Autodesk Inventor part; units mm, degrees
ref_plane "YZ Plane" through (0, 0, 0) normal (1, 0, 0) x (0, 1, 0)
ref_plane "XZ Plane" through (0, 0, 0) normal (0, 1, 0) x (-1, 0, 0)
ref_plane "XY Plane" through (0, 0, 0) normal (0, 0, 1) x (1, 0, 0)
sketch "Sketch1" plane through (0, 0, 0) normal (0, 1, 0) x (-1, 0, 0)
  line L0 (0, 0) -> (12.3, 0)
  line L1 (12.3, 0) -> (12.3, 15)
  line L2 (12.3, 15) -> (0, 15)
  line L3 (0, 15) -> (0, 0)
  dimension "d0" = 15
  dimension "d1" = 12.3
extrude "Extrusion1" add sketch "Sketch1" along normal mid plane 65
sketch "Sketch2" plane through (-12.3, -32.5, 15) normal (-1, 0, 0) x (0, 0, 1)
  circle A0 centre (-7.5, 7.5) radius 3.25
  circle A1 centre (-7.5, 57.5) radius 3.25
  circle A2 centre (-7.5, 7.5) radius 5.5
  circle A3 centre (-7.5, 57.5) radius 5.5
  line L0 (0, 0) -> (-15, 0)
  line L1 (-15, 32.5) -> (12.3047, 32.5) construction
  dimension "d4" = 6.5
  dimension "d5" = 6.5
  dimension "d8" = 11
  dimension "d9" = 11
  dimension "d26" = 25
  dimension "d27" = 25
extrude "Extrusion2" cut sketch "Sketch2" against normal through all contours A0 | A1
extrude "Extrusion3" cut sketch "Sketch2" against normal blind 21.3
sketch "Sketch3" plane through (-12.3, -32.5, 15) normal (-1, 0, 0) x (0, 0, 1)
  circle A0 centre (-7.5, 16.395) radius 3
  line L0 (0, 0) -> (-15, 0)
  circle A1 centre (-7.5, 41.395) radius 3
  point P0 (-15, 32.5)
  dimension "d14" = 6
  dimension "d22" = 16.395
  dimension "d23" = 6
  dimension "d24" = 25
hole "Hole1" at (-12.3, -16.105, 7.5) at (-12.3, 8.895, 7.5) direction (1, 0, 0) diameter 4.917 depth 15.1 tip angle 118
sketch "Sketch4" plane through (-12.3, -32.5, 15) normal (-1, 0, 0) x (0, 0, 1)
  point P0 (-15, 32.5)
properties part number "HeadbarHolderBracket_v2" material "Aluminum 6061"
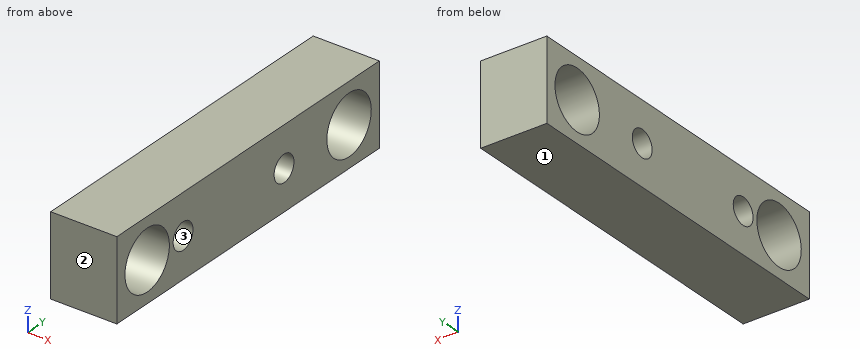
Check sheet for the modelled part. Datum: model origin and axes. Units: mm. Face numbers are marked on the shaded views. Give positions to 0.01 mm unless a question says otherwise; leave off trailing zeros. Order: outer loops, then holes, each group sorted by start corner. A loop starts at its lowest first (then second) coordinate and runs counter-clockwise, first axis right, second up. Notation, with made-up numbers: M 74,84.5 L 94,84.5 A17 cw 94,101.5 Z; hole C -4,85.5 d2. An arc over 180 degrees is marked long. Answer as CSV lines item,"result". Start each with the question number.
Item 1: Thickness scan on line 1 (Y direction, x = -9.5, z = 7.5); line 2 (Y direction, x = -10.5, z = 12.25); line 3 (Y direction, x = -2.5, z = 5.75). Record the ranges inside material, lowest first. Write a range as [from, to].
Item 2: Cross-section at A-A on z = 7.5. Enter the section's corners in (x, y).
Item 3: Cross-section at C-C on z = 11.5. Enter the section's corners in (x, y).
Item 4: Cross-section at D-D on x = -2. Enter the section's corners in (y, z) (1 decimal), plus the area to 3 significant figures.
Item 5: Mould release check, pull along Y, two halves, no side actions. Record for the marked faces 1, 2 and 3: +Y half, -Y half, draft (parallel to the pull), parting line (faces both ways), or undercut.
Item 6: Cross-section at B-B on y = 25. Enter the section's corners in (x, z).
Established:
1,line 1,"y = [-32.5, -30.5], [-19.5, -18.56], [-13.65, 6.44], [11.35, 19.5], [30.5, 32.5]"
1,line 2,"y = [-32.5, -27.77], [-22.23, 22.23], [27.77, 32.5]"
1,line 3,"y = [-32.5, -30.21], [-19.79, -17.83], [-14.38, 7.17], [10.62, 19.79], [30.21, 32.5]"
2,outline,"M -12.3,-32.5 L 0,-32.5 L 0,-30.5 L -12.3,-30.5 Z; M -12.3,-19.5 L 0,-19.5 L 0,-18.56 L -12.3,-18.56 Z; M -12.3,-13.65 L 0,-13.65 L 0,6.44 L -12.3,6.44 Z; M -12.3,11.35 L 0,11.35 L 0,19.5 L -12.3,19.5 Z; M -12.3,30.5 L 0,30.5 L 0,32.5 L -12.3,32.5 Z"
3,outline,"M -12.3,-32.5 L 0,-32.5 L 0,-28.77 L -12.3,-28.77 Z; M -12.3,-21.23 L 0,-21.23 L 0,21.23 L -12.3,21.23 Z; M -12.3,28.77 L 0,28.77 L 0,32.5 L -12.3,32.5 Z"
4,outline,"M -32.5,0 L 32.5,0 L 32.5,15 L -32.5,15 Z; hole C -25,7.5 d11; hole C -16.1,7.5 d4.9; hole C 8.9,7.5 d4.9; hole C 25,7.5 d11"
4,area,"747 mm^2"
5,face 1,"draft"
5,face 2,"-Y half"
5,face 3,"undercut"
6,outline,"M -12.3,0 L 0,0 L 0,2 L -12.3,2 Z; M -12.3,13 L 0,13 L 0,15 L -12.3,15 Z"
